Read the model definition and answer for the solid it produces. Units are mm, in the model's axes. A direction names the side the tool comes from. Coordinates: 2 decimals unless noted, no trailing zeros. Write each loop counter-clockwise with the first axis right and the second up, starting at its lowest first coordinate (ties: lowest second). Pieces come first, ordered by that corner, then holes.
Item 1: Section B-B (y = 4.5) is taken. Give the vertices of the cut face in (x, z), then the cut area to 3 significant figures.
Item 2: A tool of negligible diameter and unlimited length cuts with its end or side. For faces 1 (the face through (0, 5, 52)), 2 (the face through (30, 29, 0)), 3 (the face through (4, 29, 0)), 4 (the face through (0, 0, -1)), 5 (the face through (20, 33, -24)), from which of +Z, -Z, +X, -X, +Y, -Y can it reach the whole face along a straight path? Write none if from no direction.
Item 3: Straight lines are drawn through the part: probe 1 along X at (y, z) = (3, 36); probe 2 along Z at (x, y) = (10, 33); probe 3 along Y at (x, z) = (-0.5, -11). For each, find the intervals that lie inside material, in ascending order.
Item 4: Each of these flat-tipped pins is pushed along its axis until it touches: P1, Ø4, axis at y = 13.5, z = -23, coming from the +X side; P2, Ø14.5, axis at x = 24, z = 8.5, coming from the -Y side; P3, Ø12, axis at y = 30, z = 28.5, coming from the -X side; P4, Ø6, axis at x = 20.5, y = 11, coming from the -Z side. Where does it stop, or does it pass through?
Item 5: Section D-D (z = 38) is taken. Give the vertices of the cut face in (x, y).
Item 6: Section A-A (x = 0) is taken. Give the vertices of the cut face in (y, z), then the cut area to 3 significant figures.
Item 7: Section C-C (z = -12.5) is taken. Give the vertices of the cut face in (x, y).
Item 8: Determine the mould class of faces 6 (the face through (-4.868, 4.93, -42.349)), 7 (the face through (20, 33, 24)), 8 (the face through (45, 38, 0)) for opening direction Z: released by +Z, released by -Z, zero draft, split by the parting line, or undercut.
from build123d import *

# Parameters (mm, degrees)
SKETCH2_R                = 16
SKETCH2_R_2              = 8
BOSS_EXTRUDE1_DEPTH      = 10
BOSS_EXTRUDE2_DEPTH      = 24
BOSS_EXTRUDE2_DEPTH_BACK = 24


with BuildPart() as part:
    # Sketch2 → Boss-Extrude1 (new body)
    # profile 1 of 4: a face of its own
    with BuildSketch(Plane(origin=(0, 0, 0), x_dir=(1, 0, 0), z_dir=(0, 1, 0))):
        with Locations((0, 36)):
            Circle(SKETCH2_R)
        with Locations(Location((0, 36, 0), (0, 0, 270))):
            Circle(SKETCH2_R_2, mode=Mode.SUBTRACT)
    # profile 2 of 4: a face of its own
    with BuildSketch(Plane(origin=(0, 0, 0), x_dir=(1, 0, 0), z_dir=(0, 1, 0))):
        with BuildLine():
            Line((16, 0), (-16, 0))
            Line((-16, 0), (-16, -36))
            ThreePointArc((-16, -36), (0, -20), (16, -36))
            Line((16, -36), (16, 0))
        make_face()
    # profile 3 of 4: a face of its own
    with BuildSketch(Plane(origin=(0, 0, 0), x_dir=(1, 0, 0), z_dir=(0, 1, 0))):
        with BuildLine():
            ThreePointArc((16, 36), (0, 20), (-16, 36))
            Line((-16, 36), (-16, 0))
            Line((-16, 0), (16, 0))
            Line((16, 0), (16, 36))
        make_face()
    # profile 4 of 4: a face of its own
    with BuildSketch(Plane(origin=(0, 0, 0), x_dir=(1, 0, 0), z_dir=(0, 1, 0))):
        with Locations((0, -36)):
            Circle(SKETCH2_R)
        with Locations(Location((0, -36, 0), (0, 0, 270))):
            Circle(SKETCH2_R_2, mode=Mode.SUBTRACT)
    extrude(amount=BOSS_EXTRUDE1_DEPTH)

    # Sketch3 → Boss-Extrude2 (add, two sides: drawn at the far end of the back side and taken through both)
    with BuildSketch(Plane.XY.offset(-BOSS_EXTRUDE2_DEPTH_BACK)):
        Polygon((16, 10), (16, 29), (45, 29), (45, 48), (4, 48), (4, 10), align=None)
    extrude(amount=BOSS_EXTRUDE2_DEPTH + BOSS_EXTRUDE2_DEPTH_BACK)


solid = part.part
Established:
1. outline: (-16, -36) arc R16 ccw to (16, -36) - (16, 36) arc R16 ccw to (-16, 36) - close; hole circle Ø16 at (0, -36); hole circle Ø16 at (0, 36)
1. area: 2,710 mm2
2. face 1: +Z, +Y, -Y
2. face 2: +Z, -Z, +X, -Y
2. face 3: +Z, -Z, -X, +Y
2. face 4: +Z, -Z, +X, -X, -Y
2. face 5: -Z, +X, -X, +Y
3. probe 1: x = -16 to -8, 8 to 16
3. probe 2: z = -24 to 24
3. probe 3: y = 0 to 10
4. P1: stops at x = 16
4. P2: stops at y = 29
4. P3: stops at x = 4
4. P4: passes through
5. outline: (-15.87, 0) - (-7.75, 0) - (-7.75, 10) - (-15.87, 10) - close; (7.75, 0) - (15.87, 0) - (15.87, 10) - (7.75, 10) - close
6. outline: (0, -52) - (10, -52) - (10, -44) - (0, -44) - close; (0, -28) - (10, -28) - (10, 28) - (0, 28) - close; (0, 44) - (10, 44) - (10, 52) - (0, 52) - close
6. area: 720 mm2
7. outline: (-16, 0) - (16, 0) - (16, 29) - (45, 29) - (45, 48) - (4, 48) - (4, 10) - (-16, 10) - close
8. face 6: undercut
8. face 7: released by +Z
8. face 8: zero draft
